```python
from build123d import *

# Parameters (mm, degrees)
CROQUIS1_R              = 11
CROQUIS1_R_2            = 1.75
SALIENTE_EXTRUIR1_DEPTH = 7
CROQUIS2_R              = 3
CORTAR_EXTRUIR1_DEPTH   = 4
CROQUIS3_W              = 7
CROQUIS3_H              = 68.5
SALIENTE_EXTRUIR2_DEPTH = 10.2
CROQUIS4_R              = 2.1
CORTAR_EXTRUIR2_DEPTH   = 7


with BuildPart() as part:
    # Croquis1 → Saliente-Extruir1 (new body)
    with BuildSketch(Plane.XY):
        Polygon((17.25, -21.9), (20.25, -18.9), (20.25, 18.9), (17.25, 21.9), (-20.25, 21.9), (-20.25, -21.9), align=None)
        Circle(CROQUIS1_R, mode=Mode.SUBTRACT)
        with Locations((15.450283169, 15.450283169)):
            Circle(CROQUIS1_R_2, mode=Mode.SUBTRACT)
        with Locations((15.450283169, -15.450283169)):
            Circle(CROQUIS1_R_2, mode=Mode.SUBTRACT)
        with Locations((-15.450283169, -15.450283169)):
            Circle(CROQUIS1_R_2, mode=Mode.SUBTRACT)
        with Locations((-15.450283169, 15.450283169)):
            Circle(CROQUIS1_R_2, mode=Mode.SUBTRACT)
    extrude(amount=SALIENTE_EXTRUIR1_DEPTH)

    # Croquis2 → Cortar-Extruir1 (cut)
    with BuildSketch(Plane.XY.offset(7)):
        with Locations((15.450283169, 15.450283169)):
            Circle(CROQUIS2_R)
        with Locations((15.450283169, -15.450283169)):
            Circle(CROQUIS2_R)
        with Locations((-15.450283169, -15.450283169)):
            Circle(CROQUIS2_R)
        with Locations((-15.450283169, 15.450283169)):
            Circle(CROQUIS2_R)
    extrude(amount=-CORTAR_EXTRUIR1_DEPTH, mode=Mode.SUBTRACT)

    # Croquis3 → Saliente-Extruir2 (add)
    with BuildSketch(Plane(origin=(0, 0, 0), x_dir=(-1, 0, 0), z_dir=(0, 0, -1))):
        with Locations((23.75, 0)):
            Rectangle(CROQUIS3_W, CROQUIS3_H)
    extrude(amount=-SALIENTE_EXTRUIR2_DEPTH)

    # Croquis4 → Cortar-Extruir2 (cut)
    with BuildSketch(Plane.ZY.offset(27.25)):
        with Locations((5.1, 28.15)):
            Circle(CROQUIS4_R)
        with Locations((5.1, -28.15)):
            Circle(CROQUIS4_R)
    extrude(amount=-CORTAR_EXTRUIR2_DEPTH, mode=Mode.SUBTRACT)


solid = part.part
```
Build history of the part. All positions in model axes, mm. A direction names the side the tool comes from. Round coordinates to 2 decimals unless told otherwise and drop trailing zeros. Loops run counter-clockwise (first coordinate to the right, second up) from the corner with the lowest first, then second, coordinate; pieces in that order, holes last. Notation, with made-up numbers: M 31,-38.5 L 39,-38.5 A18 ccw 39,-33.5 Z; hole C 7,26 d10. An arc over 180 degrees is marked long. Answer as CSV lines item,"result".
1. Cut at B-B on z = 5.1. Write the cut outline in (x, y), then the cut area to 3 significant figures.
Resolved:
outline,"M -27.25,-34.25 L -20.25,-34.25 L -20.25,-30.25 L -27.25,-30.25 Z; M -27.25,-26.05 L -20.25,-26.05 L -20.25,-21.9 L 17.25,-21.9 L 20.25,-18.9 L 20.25,18.9 L 17.25,21.9 L -20.25,21.9 L -20.25,26.05 L -27.25,26.05 Z; M -27.25,30.25 L -20.25,30.25 L -20.25,34.25 L -27.25,34.25 Z; hole C -15.45,-15.45 d6; hole C -15.45,15.45 d6; hole C 0,0 d22; hole C 15.45,-15.45 d6; hole C 15.45,15.45 d6"
area,"1,690 mm²"
2. Flat gauge pins, fed straight in: P1, Ø3, axis at x = -15.45, y = -15.45, coming from the +Z side; P2, Ø9.5, axis at x = 15.45, y = 15.45, coming from the +Z side; P3, Ø1.8, axis at x = -15, y = 14, coming from the +Z side; P4, Ø3, axis at y = -25.5, z = 9, coming from the +X side. Where does each tip first touch, or does it go through?
Resolved:
P1,"passes through"
P2,"stops at z = 7"
P3,"stops at z = 3"
P4,"stops at x = -20.25"
3. Cut at C-C on y = -28.15. Write the cut outline in (x, z), then the cut area to 3 significant figures.
Resolved:
outline,"M -27.25,0 L -20.25,0 L -20.25,3 L -27.25,3 Z; M -27.25,7.2 L -20.25,7.2 L -20.25,10.2 L -27.25,10.2 Z"
area,"42.0 mm²"
4. 3-axis set-ups, long thin cutter, end or side, ignore diameter. For faces 1 (the flat face through (-1, 21.9, 3)), 2 (the flat face through (-14, 14, 3)), 3 (the flat face through (-2, -21.9, 3)): which of +Z, -Z, +X, -X, +Y, -Y reach the whole face in a straight line?
Resolved:
face 1,"+Z, -Z, +X, +Y"
face 2,"+Z"
face 3,"+Z, -Z, +X, -Y"
5. Two-plate mould, pull along X, no slides. Class faces 4 (the cylindrical face through (13.24, 17.48, 5.03)), 5 (the flat face through (-27.25, 0, 5)), 6 (the flat face through (-14, -17, 3)), 7 (the flat face through (-24, 34.25, 5)): released by +X, released by -X, zero draft, split by the parting line, or undercut.
Resolved:
face 4,"undercut"
face 5,"released by -X"
face 6,"undercut"
face 7,"zero draft"
6. Wall check: probe 1 along Y at (x, z) = (-22, 5.1); probe 2 along Y at (x, z) = (-16, 6.5); probe 3 along Z at (x, y) = (-11, 10). Give the ranges that are in metal, low to high. Write a range as [from, to].
Resolved:
probe 1,"y = [-34.25, -30.25], [-26.05, 26.05], [30.25, 34.25]"
probe 2,"y = [-21.9, -18.4], [-12.5, 12.5], [18.4, 21.9]"
probe 3,"z = [0, 7]"
7. Cut at A-A on x = 0. Write the cut outline in (y, z), then the cut area to 3 significant figures.
Resolved:
outline,"M -21.9,0 L -11,0 L -11,7 L -21.9,7 Z; M 11,0 L 21.9,0 L 21.9,7 L 11,7 Z"
area,"153 mm²"
8. Cut at D-D on x = -22. Write the cut outline in (y, z), then the cut area to 3 significant figures.
Resolved:
outline,"M -34.25,0 L 34.25,0 L 34.25,10.2 L -34.25,10.2 Z; hole C -28.15,5.1 d4.2; hole C 28.15,5.1 d4.2"
area,"671 mm²"
